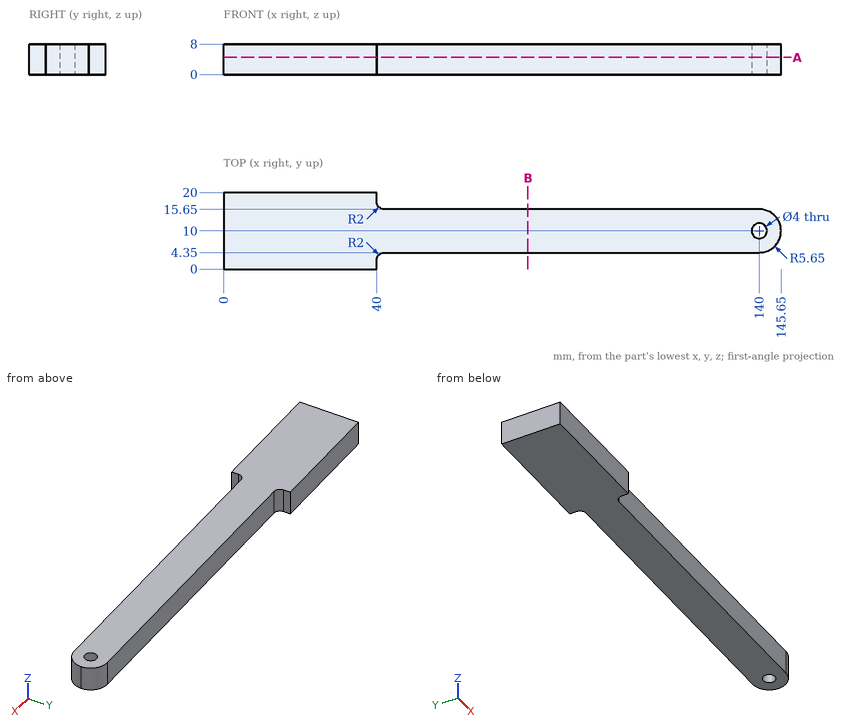
Input: dimensioned drawing with shaded views. Units: mm. Origin: part minimum x, y, z. Round coordinates to 2 decimals unless told otherwise and drop trailing zeros. Write each loop counter-clockwise with the first axis right and the second up, starting at its lowest first coordinate (ties: lowest second). Pieces come first, ordered by that corner, then holes. Notation, with made-up numbers: (61.5, 35.5) -> (108.5, 35.5) arc R29 cw to (108.5, 72.5) -> close; hole circle Ø8 at (48.25, 0.5). An arc over 180 degrees is marked (long way). Use CSV: the item, a comma, the result in double quotes. Start each with the question number.
Q1. Section A-A (z = 4.5). Return loops of the section in (x, y).
Q2. Line query: L1, parallel to Y at x = 140, z = 1.75; L2, parallel to Y at x = 54, z = 0.5; L3, parallel to X at y = 2.5, z = 7.25. Output: solid intervals per line, ascending.
Q3. Section B-B (x = 79.5). Return loops of the section in (y, z).
Q4. First-contact query: pin 1 Ø2 at (x, z) = (33, 6.5) entering from -Y; pin 2 Ø1.2 at (y, z) = (1, 5.5) entering from +X; pin 3 Ø2.5 at (x, z) = (92.5, 5.5) entering from -Y. Flat tips, straight axial feed; report the tip coordinate or a pass-through.
Result sheet:
1,outline,"(0, 0) -> (40, 0) -> (40, 2.35) arc R2 cw to (42, 4.35) -> (140, 4.35) arc R5.65 ccw to (145.65, 10) arc R5.65 ccw to (140, 15.65) -> (42, 15.65) arc R2 cw to (40, 17.65) -> (40, 20) -> (0, 20) -> close; hole circle Ø4 at (140, 10)"
2,L1,"4.35 to 8, 12 to 15.65"
2,L2,"4.35 to 15.65"
2,L3,"0 to 40.01"
3,outline,"(4.35, 0) -> (15.65, 0) -> (15.65, 8) -> (4.35, 8) -> close"
4,pin 1,"y = 0"
4,pin 2,"x = 40"
4,pin 3,"y = 4.35"
